Autodesk Inventor part; units mm, degrees
ref_plane "YZ Plane" through (0, 0, 0) normal (1, 0, 0) x (0, 1, 0)
ref_plane "XZ Plane" through (0, 0, 0) normal (0, 1, 0) x (-1, 0, 0)
ref_plane "XY Plane" through (0, 0, 0) normal (0, 0, 1) x (1, 0, 0)
sketch "Sketch1" plane through (0, 0, 0) normal (0, 0, 1) x (1, 0, 0)
  circle A0 centre (0, 0) radius 6
  dimension "d0" = 12
extrude "Extrusion1" add sketch "Sketch1" along normal blind 30.5
sketch "Sketch2" plane through (0, 0, 30.5) normal (0, 0, 1) x (1, 0, 0)
  circle A0 centre (-0.8, 0) radius 0.75
  circle A1 centre (0.8, 0) radius 0.75
  circle A2 centre (0, 0) radius 1.75
  dimension "d3" = 1.5
  dimension "d4" = 1.5
  dimension "d5" = 1.6
  dimension "d6" = 0.8
  dimension "d7" = 3.5
extrude "Extrusion2" add sketch "Sketch2" along normal blind 30 contours A0 | A1
sketch "Sketch3" plane through (0, 0, 0) normal (0, 0, -1) x (-1, 0, 0)
  circle A0 centre (0, 0) radius 4.4
  dimension "d10" = 8.8
extrude "Extrusion3" add sketch "Sketch3" along normal blind 4
sketch "Sketch4" plane through (0, 0, -4) normal (0, 0, -1) x (-1, 0, 0)
  circle A0 centre (0, 0) radius 2.5
  dimension "d13" = 5
extrude "Extrusion4" cut sketch "Sketch4" against normal blind 2
chamfer "Chamfer1" distance 1 angle 45 1 edges at (2.5, 0, -4)
thread "Thread1"
fillet "Fillet1" radius 0.4 2 edges at (-6, 0, 30.5) (-6, 0, 0)
properties part number "COTS_GENERIC_Engraving_laser"
CAD build for the part. Positions are in the model's coordinates, mm. A direction names the side the tool comes from. Give positions to 0.01 mm unless a question says otherwise; leave off trailing zeros. Order: outer loops, then holes, each group sorted by start corner. A loop starts at its lowest first (then second) coordinate and runs counter-clockwise, first axis right, second up.
(1) Mould opens along X. For faces 1 (the cylindrical face through (-1.55, -0.03, 45.29)), 2 (the flat face through (0, -5, 0)), 3 (the cylindrical face through (-6, 0, 15)) say: released by +X, released by -X, zero draft, split by the parting line, or undercut.
(2) Saw through at A-A, the plane y = 0. Give the cut face in (x, z).
(3) Flat gauge pins, fed straight in: pin 1 (2 mm diameter, centred on x = 0.5, z = 45, fed in from +Y); pin 2 (3 mm diameter, centred on y = 3.5, z = 9, fed in from +X); pin 3 (5 mm diameter, centred on x = 2.5, z = 8, fed in from -Y); pin 4 (2 mm diameter, centred on x = -2.5, z = 29.5, fed in from -Y). Where does each tip first touch, or does it go through?
(4) Drill centre lines: L1, parallel to Y at x = 0, z = -2.55; L2, parallel to Z at x = -0.5, y = 4; L3, parallel to Z at x = 5.5, y = -0.25. Where is each one in solid material? Low to high.
(5) Saw through at B-B, the plane z = 41.5. Give the cut face in (x, y), then the cut area to 3 significant figures.
(6) Saw through at C-C, the plane z = 9. Give the cut face in (x, y), then the cut area to 3 significant figures.
(7) Tool access for faces 4 (the cylindrical face through (1.515, -0.225, 45.29)), 5 (the cylindrical face through (-4.197, -1.322, -1.972)), 6 (the flat face through (1, 0, 60.5)): list every direction of +Z, -Z, +X, -X, +Y, -Y with a clear straight run to the whole face (end or side of a thin tool).
Results found:
1. face 1: undercut
1. face 2: zero draft
1. face 3: split by the parting line
2. outline: (-6, 0.4) arc R0.4 ccw to (-5.6, 0) - (-4.4, 0) - (-4.4, -4) - (-3.5, -4) - (-2.5, -3) - (-2.5, -2) - (2.5, -2) - (2.5, -3) - (3.5, -4) - (4.4, -4) - (4.4, 0) - (5.6, 0) arc R0.4 ccw to (6, 0.4) - (6, 30.1) arc R0.4 ccw to (5.6, 30.5) - (1.55, 30.5) - (1.55, 60.5) - (0.05, 60.5) - (0.05, 30.5) - (-0.05, 30.5) - (-0.05, 60.5) - (-1.55, 60.5) - (-1.55, 30.5) - (-5.6, 30.5) arc R0.4 ccw to (-6, 30.1) - close
3. pin 1: stops at y = 0.75
3. pin 2: stops at x = 5.66
3. pin 3: stops at y = -6
3. pin 4: stops at y = -5.81
4. L1: y = -4.4 to -2.5, 2.5 to 4.4
4. L2: z = -4 to 30.5
4. L3: z = 0 to 30.5
5. outline: circle Ø1.5 at (-0.8, 0); circle Ø1.5 at (0.8, 0)
5. area: 3.53 mm2
6. outline: circle Ø12 at (0, 0)
6. area: 113 mm2
7. face 4: +Z
7. face 5: -Z
7. face 6: +Z, +X, -X, +Y, -Y
